Geometry: see drawing. Coordinates: mm, zero at the bounding-box minimum. Coordinates: 2 decimals unless noted, no trailing zeros. Order: outer loops, then holes, each group sorted by start corner. A loop starts at its lowest first (then second) coordinate and runs counter-clockwise, first axis right, second up. Notation, with made-up numbers: M -12.75,-17.5 L -2.75,-17.5 A35 ccw -2.75,16.5 Z; hole C 7.5,20 d2. An arc over 180 degrees is marked long. One line per item, written item: value.
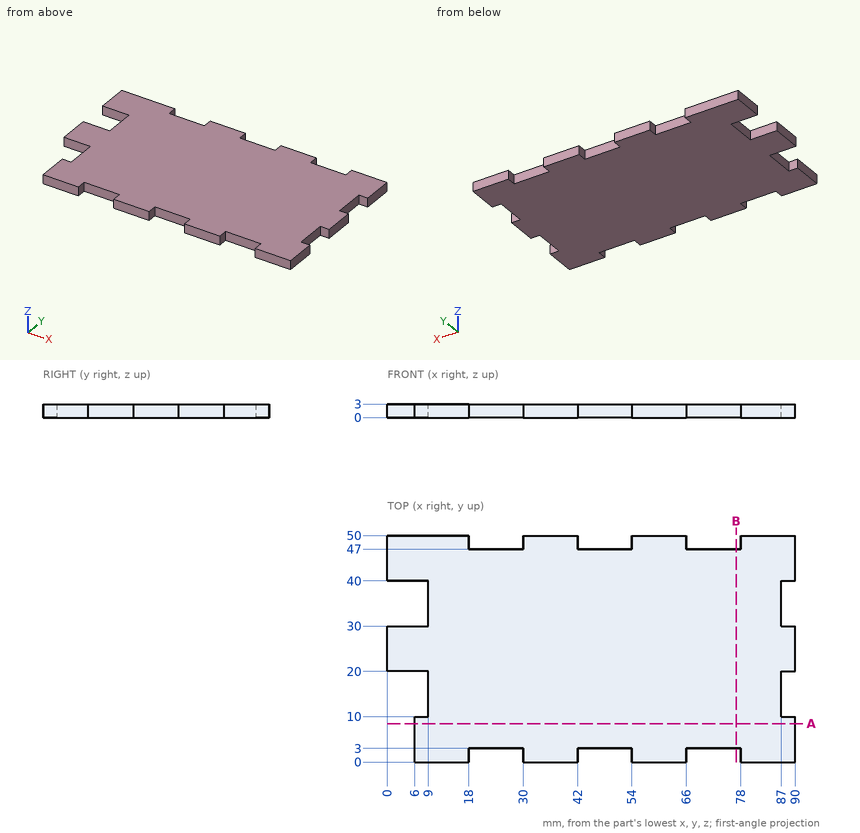
(1) First-contact query: pin 1 (1.5 mm diameter, centred on x = 45.5, z = 1.5, fed in from +Y); pin 2 (0.9 mm diameter, centred on y = 37, z = 1.5, fed in from +X); pin 3 (1.5 mm diameter, centred on x = 49, z = 1, fed in from -Y). Flat tips, straight axial feed; report the tip coordinate or a pass-through.
Data:
pin 1: stops at y = 47
pin 2: stops at x = 87
pin 3: stops at y = 3
(2) Cut plane A-A on y = 8.5. Output: boundary loops of the cut face in (x, z).
Data:
outline: M 6,0 L 90,0 L 90,3 L 6,3 Z
(3) Cut plane B-B on x = 77. Output: boundary loops of the cut face in (y, z), plus the area to 3 significant figures.
Data:
outline: M 3,0 L 47,0 L 47,3 L 3,3 Z
area: 132 mm2
(4) Ray query, line 1 (X direction, y = 48, z = 0.4); line 2 (Y direction, x = 74.5, z = 0.8); line 3 (X direction, y = 13.5, z = 1.35). Return the intervals inside material, ascending. Write a range as from..to.
Data:
line 1: x = 0..18, 30..42, 54..66, 78..90
line 2: y = 3..47
line 3: x = 9..87
